Can you work these out from the model? Positions are in its coordinate system, mm. A direction names the side the tool comes from. Round coordinates to 2 decimals unless told otherwise and drop trailing zeros. Write each loop counter-clockwise with the first axis right and the second up, starting at its lowest first coordinate (ties: lowest second). Pieces come first, ordered by that corner, then holes. Notation, with made-up numbers: M 62.5,23.25 L 69.5,23.25 A19 cw 69.5,36.25 Z; hole C 1,69.25 d5. An arc over 180 degrees is marked long. Answer in a Markdown table with one row per item. Add a question column.
(1) Suppose I cut it at C-C, the plane x = 0. Count the separate pieces of the cut face and the enclosed holes in it, then the cut area to 3 significant figures.
(2) For faces 5 (the face through (-10.16, -3, 0)), 6 (the face through (0.549, -18.044, 11.412)), which set-ups out of +Z, -Z, +X, -X, +Y, -Y let a thin tool reach every point of the face, with its end or its side?
(3) Suppose I cut it at B-B, the plane y = -4.5. Write out the boundary of the cut face in (x, z) (3 decimals), then the cut area to 3 significant figures.
(4) If I drill on probe 1 along Y at (x, z) = (0, -11.7) (3 decimals); probe 2 along Z at (x, y) = (9.75, -175); probe 3 along X at (y, z) = (-133.5, -7.25), over which ranges is the centre line in solid material (lowest first)?
(5) I'm going to push flat-ended pins straight in: pin 1 (1.5 mm diameter, centred on x = -7, z = 8.5, fed in from +Y); pin 2 (11 mm diameter, centred on x = 0, y = -22.225, fed in from -Z). Where does each tip first touch, or does it pass through?
(6) Suppose I cut it at A-A, the plane z = 5.5. Write out the boundary of the cut face in (x, y) (3 decimals), then the cut area to 3 significant figures.
(7) If we mould it in two halves opening along X, with no side actions, what happens to faces 1 (the face through (0.91, -115.24, 11.41)), 2 (the face through (12.7, -3, 0)), 3 (the face through (0.549, -195.844, -11.448)), 4 (the face through (11, 220.345, 0))? For each: released by +X, released by -X, zero draft, split by the parting line, or undercut.
from build123d import *

# Parameters (mm, degrees)
F0_W     = 25.4
F0_H     = 25.4
F1_DEPTH = 220.345
F2_R     = 3.175
F3_T     = -2.54
F5_D     = 8.4328


with BuildPart() as f1:
    # F0 (on Front) → F1 (new body, symmetric)
    with BuildSketch(Plane.XZ):
        Rectangle(F0_W, F0_H)
    extrude(amount=F1_DEPTH, both=True)

    # F2
    f2_edges = [f1.edges().sort_by_distance(p)[0] for p in [
        (-12.7, 0, 12.7),
        (12.7, 0, 12.7),
        (-12.7, 0, -12.7),
        (12.7, 0, -12.7),
    ]]
    fillet(f2_edges, radius=F2_R)

    # F3
    f3_openings = [f1.faces().sort_by_distance(p)[0] for p in [
        (0, -220.345, 0),
        (0, 220.345, 0),
    ]]
    offset(amount=F3_T, openings=f3_openings)

    # F5 (through all)
    with Locations(Plane.XY.offset(12.7)):
        with Locations((0, -200.025), (0, -22.225), (0, 200.025), (0, -111.125)):
            Hole(F5_D / 2)


solid = f1.part
Calculated:
| question | item | result |
|---|---|---|
| 1 | separate pieces | 10 |
| 1 | enclosed holes | 0 |
| 1 | area | 2,070 mm² |
| 2 | face 5 | +Y, -Y |
| 2 | face 6 | +Z, -Z |
| 3 | outline | M -12.7,-9.525 A3.175 ccw -9.525,-12.7 L 9.525,-12.7 A3.175 ccw 12.7,-9.525 L 12.7,9.525 A3.175 ccw 9.525,12.7 L -9.525,12.7 A3.175 ccw -12.7,9.525 Z; hole M -10.16,-9.525 A0.635 ccw -9.525,-10.16 L 9.525,-10.16 A0.635 ccw 10.16,-9.525 L 10.16,9.525 A0.635 ccw 9.525,10.16 L -9.525,10.16 A0.635 ccw -10.16,9.525 Z |
| 3 | area | 224 mm² |
| 4 | probe 1 | -220.345 to -204.241, -195.809 to -115.341, -106.909 to -26.441, -18.009 to 195.809, 204.241 to 220.345 |
| 4 | probe 2 | -12.69 to -10.12, 10.12 to 12.69 |
| 4 | probe 3 | -12.7 to -10.16, 10.16 to 12.7 |
| 5 | pin 1 | through |
| 5 | pin 2 | z = -12.7 |
| 6 | outline | M -12.7,-220.345 L -10.16,-220.345 L -10.16,220.345 L -12.7,220.345 Z; M 10.16,-220.345 L 12.7,-220.345 L 12.7,220.345 L 10.16,220.345 Z |
| 6 | area | 2,240 mm² |
| 7 | face 1 | undercut |
| 7 | face 2 | released by +X |
| 7 | face 3 | undercut |
| 7 | face 4 | zero draft |
